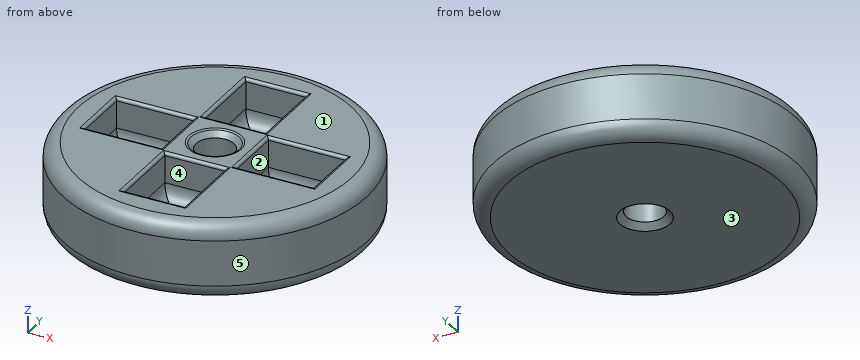
from build123d import *

# Parameters (mm, degrees)
F0_R     = 12.7
F1_DEPTH = 6.35
F2_R     = 1.5875
F3_DEPTH = 25.4
F4_R     = 1.27
F5_SIZE  = 0.508
F6_W     = 2.54
F6_H     = 6.477
F6_W_2   = 6.477
F6_H_2   = 5.08
F6_W_3   = 5.08
F7_DEPTH = 3.81
F8_R     = 1.27
F9_R     = 0.254


with BuildPart() as f1:
    # F0 (on Top) → F1 (new body)
    with BuildSketch(Plane.XY):
        Circle(F0_R)
    extrude(amount=F1_DEPTH)

    # F2 (on face) → F3 (cut)
    with BuildSketch(Plane.XY.offset(6.35)):
        Circle(F2_R)
    extrude(amount=-F3_DEPTH, mode=Mode.SUBTRACT)

    # F4
    f4_edges = [f1.edges().sort_by_distance(p)[0] for p in [
        (12.7, 0, 3.175),
        (-12.7, 0, 0),
        (-12.7, 0, 6.35),
    ]]
    fillet(f4_edges, radius=F4_R)

    # F5
    f5_edges = [f1.edges().sort_by_distance(p)[0] for p in [
        (-1.5875, 0, 6.35),
        (-1.5875, 0, 0),
    ]]
    chamfer(f5_edges, length=F5_SIZE)

    # F6 (on face) → F7 (cut)
    with BuildSketch(Plane.XY.offset(6.35)):
        with Locations((-1.27, 6.35)):
            Rectangle(F6_W, F6_H)
        with Locations((1.27, 6.35)):
            Rectangle(F6_W, F6_H)
        with Locations((-6.35, 0)):
            Rectangle(F6_W_2, F6_H_2)
        with Locations((0, -6.35)):
            Rectangle(F6_W_3, F6_H)
        with Locations((6.35, 0)):
            Rectangle(F6_W_2, F6_H_2)
    extrude(amount=-F7_DEPTH, mode=Mode.SUBTRACT)

    # F8
    f8_edges = [f1.edges().sort_by_distance(p)[0] for p in [
        (-2.54, -6.35, 2.54),
        (0, -9.5885, 2.54),
        (2.54, -6.35, 2.54),
        (0, -3.1115, 2.54),
        (6.35, -2.54, 2.54),
        (9.5885, 0, 2.54),
        (6.35, 2.54, 2.54),
        (3.1115, 0, 2.54),
        (-6.35, 2.54, 2.54),
        (-9.5885, 0, 2.54),
        (-6.35, -2.54, 2.54),
        (-3.1115, 0, 2.54),
        (0, 3.1115, 2.54),
        (2.54, 6.35, 2.54),
        (0, 9.5885, 2.54),
        (-2.54, 6.35, 2.54),
    ]]
    fillet(f8_edges, radius=F8_R)

    # F9
    f9_edges = [f1.edges().sort_by_distance(p)[0] for p in [
        (-11.43, 0, 6.35),
        (-2.54, -6.35, 6.35),
        (0, -9.5885, 6.35),
        (2.54, -6.35, 6.35),
        (0, -3.1115, 6.35),
        (-6.35, 2.54, 6.35),
        (-9.5885, 0, 6.35),
        (-6.35, -2.54, 6.35),
        (-3.1115, 0, 6.35),
        (-2.0955, 0, 6.35),
        (6.35, -2.54, 6.35),
        (9.5885, 0, 6.35),
        (6.35, 2.54, 6.35),
        (3.1115, 0, 6.35),
        (0, 3.1115, 6.35),
        (2.54, 6.35, 6.35),
        (0, 9.5885, 6.35),
        (-2.54, 6.35, 6.35),
    ]]
    fillet(f9_edges, radius=F9_R)


solid = f1.part
The listing builds one solid part. Answer for the finished solid, in the listing's coordinates (mm). Face numbers are marked on the shaded views. A direction names the side the tool comes from. Coordinates: 2 decimals unless noted, no trailing zeros. Order: outer loops, then holes, each group sorted by start corner. A loop starts at its lowest first (then second) coordinate and runs counter-clockwise, first axis right, second up. Notation, with made-up numbers: (44.25, 62) -> (83.25, 62) arc R30 cw to (83.25, 86) -> close; hole circle Ø11 at (-39.5, 20.25). An arc over 180 degrees is marked (long way). Answer in a Markdown table with one row per item. Add a question column.
Item 1: Which of the six approach directions +Z, -Z, +X, -X, +Y, -Y give full straight-line access (tool end or side, diameter ignored) to the marked faces 1 and 2?
Item 2: Each of these flat-tipped pins is pushed along its axis until it touches: P1, Ø3, axis at x = 6.5, z = 3.5, coming from the +Y side; P2, Ø1, axis at x = -4.5, y = 6.5, coming from the -Z side; P3, Ø2, axis at x = -0.5, y = 6, coming from the +Z side; P4, Ø2.5, axis at y = -7.5, z = 5.5, coming from the +X side. Where does it stop, or does it pass through?
Item 3: Determine the mould class of the marked faces 3, 4 and 5 for opening direction X: +X half, -X half, draft (parallel to the pull), parting line (faces both ways), or undercut.
Item 4: Find section C-C (z = 4.5). Write down the section's boundary in (x, y) (1 decimal), then the cut area to 3 significant figures.
Item 5: Find the intervals of material crossed by L1, parallel to Y at x = 0, z = 3.75; L2, parallel to Y at x = 0, z = 2; L3, parallel to Y at x = -1, z = 3.75, in increasing order. Write a range as from..to.
Result set:
| question | item | result |
|---|---|---|
| 1 | face 1 | +Z, +X, -X, +Y, -Y |
| 1 | face 2 | +Z |
| 2 | P1 | stops at y = 11.67 |
| 2 | P2 | stops at z = 0 |
| 2 | P3 | stops at z = 2.56 |
| 2 | P4 | stops at x = 11.03 |
| 3 | face 3 | draft |
| 3 | face 4 | undercut |
| 3 | face 5 | parting line |
| 4 | outline | circle Ø25.4 at (0, 0); hole (-9.6, -2.5) -> (-3.1, -2.5) -> (-3.1, 2.5) -> (-9.6, 2.5) -> close; hole (-2.5, -9.6) -> (2.5, -9.6) -> (2.5, -3.1) -> (-2.5, -3.1) -> close; hole (-2.5, 3.1) -> (2.5, 3.1) -> (2.5, 9.6) -> (-2.5, 9.6) -> close; hole circle Ø3.2 at (0, 0); hole (3.1, -2.5) -> (9.6, -2.5) -> (9.6, 2.5) -> (3.1, 2.5) -> close |
| 4 | area | 367 mm² |
| 5 | L1 | y = -12.7..-9.59, -3.11..-1.59, 1.59..3.11, 9.59..12.7 |
| 5 | L2 | y = -12.7..-1.59, 1.59..12.7 |
| 5 | L3 | y = -12.66..-9.59, -3.11..-1.23, 1.23..3.11, 9.59..12.66 |
